For this review, take the finished solid that the model builds, in its own axes (mm). Give positions to 0.01 mm unless a question says otherwise; leave off trailing zeros. Write each loop counter-clockwise with the first axis right and the second up, starting at its lowest first coordinate (ties: lowest second). Pieces come first, ordered by that corner, then holes. Notation, with made-up numbers: M -5.75,64 L 18.25,64 A19 ccw 18.25,98 Z; hole C 83.5,13 d3. An arc over 180 degrees is marked long. One line per item, written item: value. Start each with the question number.
Item 1: Consider section B-B, the plane x = 0. Write out the cut boundary in (y, z), and give its area (3 significant figures).
Item 2: Clearance check with a flat-ended pin moving along its axis: pin 1 Ø4 at (x, y) = (-3, 1) entering from -Z. State where the tip first meets the part, or that it passes through.
Item 3: Consider section A-A, the plane z = 0. Write out the cut boundary in (x, y), and give its area (3 significant figures).
Item 4: Consider section D-D, the plane y = 3. Write out the cut boundary in (x, z).
Item 5: Consider section C-C, the plane y = 7.25. Write out the cut boundary in (x, z), and give its area (3 significant figures).
Item 6: To check wall thickness, follow probe 1 along Y at (x, z) = (3.5, 0.5); probe 2 along Y at (x, z) = (3, 0.25); probe 3 along Z at (x, y) = (0, 2.25). State the ranges of each line that lie inside material, in increasing order.
Solid Edge part; units mm, degrees
sketch "Sketch1" plane through (0, 0, 0) normal (0, -1, 0) x (1, 0, 0)
  circle A0 centre (0, 0) radius 4
  circle A1 centre (0, 0) radius 1
extrude "Protrusion1" add sketch "Sketch1" against normal blind 1
sketch "Sketch2" plane through (0, 1, 0) normal (0, 1, 0) x (-1, 0, 0)
  circle A0 centre (0, 0) radius 1.5
extrude "ExtrudedProtrusion_3" add sketch "Sketch2" along normal blind 3
mirror "Mirror1" about plane through (0, 4, 0) normal (0, 1, 0) of "ExtrudedProtrusion_3", "Protrusion1"
sketch "Sketch3" plane through (0, 0, 0) normal (0, -1, 0) x (1, 0, 0)
  circle A0 centre (0, 0) radius 1
extrude "ExtrudedCutout_1" cut sketch "Sketch3" against normal blind 15.8267
fillet "Round_1" radius 3 1 edges at (1.5, 1, 0)
fillet "Round_2" radius 3 1 edges at (1.5, 7, 0)
Model answer:
1. outline: M 0,-4 L 1,-4 A3 cw 3.96,-1.5 L 4.04,-1.5 A3 cw 7,-4 L 8,-4 L 8,-1 L 0,-1 Z; M 0,1 L 8,1 L 8,4 L 7,4 A3 cw 4.04,1.5 L 3.96,1.5 A3 cw 1,4 L 0,4 Z
1. area: 25.3 mm2
2. pin 1: stops at z = -3.87
3. outline: M -4,0 L -1,0 L -1,8 L -4,8 L -4,7 A3 cw -1.5,4.04 L -1.5,3.96 A3 cw -4,1 Z; M 1,0 L 4,0 L 4,1 A3 cw 1.5,3.96 L 1.5,4.04 A3 cw 4,7 L 4,8 L 1,8 Z
3. area: 25.3 mm2
4. outline: C 0,0 d3.31; hole C 0,0 d2
5. outline: C 0,0 d8; hole C 0,0 d2
5. area: 47.1 mm2
6. probe 1: y = 0 to 1.12, 6.88 to 8
6. probe 2: y = 0 to 1.35, 6.65 to 8
6. probe 3: z = -2.03 to -1, 1 to 2.03
